```python
from build123d import *

# Parameters (mm, degrees)
EXTRUDE_2_DEPTH     = 70
EXTRUDE_3_DEPTH     = 2
SKETCH_7_W          = 20
SKETCH_7_H          = 18
SKETCH_7_R          = 1.6
EXTRUDE_5_DEPTH     = 4
SKETCH_8_W          = 28
SKETCH_8_H          = 11.5
CUT_EXTRUDE_2_DEPTH = 11.5


with BuildPart() as part:
    # Sketch 1 → Extrude 2 (new body)
    with BuildSketch(Plane.ZY.offset(35)):
        with BuildLine():
            Line((-22.27263006, 25.369984756), (23.72736994, 25.369984756))
            ThreePointArc((23.72736994, 25.369984756), (31.859097923, 22.001712739), (35.22736994, 13.869984756))
            Line((35.22736994, 13.869984756), (35.22736994, 7.291341901))
            ThreePointArc((35.22736994, 7.291341901), (31.859097923, -0.840386083), (23.72736994, -4.208658099))
            Line((23.72736994, -4.208658099), (-22.27263006, -4.208658099))
            ThreePointArc((-22.27263006, -4.208658099), (-30.404358044, -0.840386083), (-33.77263006, 7.291341901))
            Line((-33.77263006, 7.291341901), (-33.77263006, 13.869984756))
            ThreePointArc((-33.77263006, 13.869984756), (-30.404358044, 22.001712739), (-22.27263006, 25.369984756))
        make_face()
        with BuildLine():
            ThreePointArc((-22.27263006, 23.869984756), (-29.343697872, 20.941052568), (-32.27263006, 13.869984756))
            Line((-32.27263006, 13.869984756), (-32.27263006, 7.291341901))
            ThreePointArc((-32.27263006, 7.291341901), (-29.343697872, 0.220274089), (-22.27263006, -2.708658099))
            Line((-22.27263006, -2.708658099), (23.72736994, -2.708658099))
            ThreePointArc((23.72736994, -2.708658099), (30.798437752, 0.220274089), (33.72736994, 7.291341901))
            Line((33.72736994, 7.291341901), (33.72736994, 13.869984756))
            ThreePointArc((33.72736994, 13.869984756), (30.798437752, 20.941052568), (23.72736994, 23.869984756))
            Line((23.72736994, 23.869984756), (-22.27263006, 23.869984756))
        make_face(mode=Mode.SUBTRACT)
    extrude(amount=-EXTRUDE_2_DEPTH)

    # Sketch 1_4 → Extrude 3 (add)
    with BuildSketch(Plane.ZY.offset(35)):
        with BuildLine():
            Line((-22.27263006, 23.869984756), (23.72736994, 23.869984756))
            ThreePointArc((23.72736994, 23.869984756), (30.798437752, 20.941052568), (33.72736994, 13.869984756))
            Line((33.72736994, 13.869984756), (33.72736994, 7.291341901))
            ThreePointArc((33.72736994, 7.291341901), (30.798437752, 0.220274089), (23.72736994, -2.708658099))
            Line((23.72736994, -2.708658099), (-22.27263006, -2.708658099))
            ThreePointArc((-22.27263006, -2.708658099), (-29.343697872, 0.220274089), (-32.27263006, 7.291341901))
            Line((-32.27263006, 7.291341901), (-32.27263006, 13.869984756))
            ThreePointArc((-32.27263006, 13.869984756), (-29.343697872, 20.941052568), (-22.27263006, 23.869984756))
        make_face()
    extrude(amount=-EXTRUDE_3_DEPTH)

    # Sketch 7 → Extrude 5 (add)
    with BuildSketch(Plane(origin=(35, 0, 0), x_dir=(0, 0, -1), z_dir=(1, 0, 0))):
        with Locations((-2.22736994, -11.708658099)):
            Rectangle(SKETCH_7_W, SKETCH_7_H)
        with Locations((4.77263006, -17.708658099)):
            Circle(SKETCH_7_R, mode=Mode.SUBTRACT)
        with Locations((-9.22736994, -17.708658099)):
            Circle(SKETCH_7_R, mode=Mode.SUBTRACT)
    extrude(amount=-EXTRUDE_5_DEPTH)

    # Sketch 8 → Cut-Extrude 2 (cut)
    with BuildSketch(Plane(origin=(0, 0, -33.77263006), x_dir=(-1, 0, 0), z_dir=(0, 0, -1))):
        with Locations((19, 1.541341901)):
            Rectangle(SKETCH_8_W, SKETCH_8_H)
    extrude(amount=-CUT_EXTRUDE_2_DEPTH, mode=Mode.SUBTRACT)


solid = part.part
```
Input: part model. Units: mm. Frame: model coordinates. A direction names the side the tool comes from. Round coordinates to 2 decimals unless told otherwise and drop trailing zeros. Loops run counter-clockwise (first coordinate to the right, second up) from the corner with the lowest first, then second, coordinate; pieces in that order, holes last. Notation, with made-up numbers: (-5, -15) -> (22, -15) arc R20 ccw to (22, 2) -> close; hole circle Ø10 at (-27.75, 8). An arc over 180 degrees is marked (long way). Write each question's results on one line, items separated by ' | '.
1. Section B-B (z = -28.5). Return loops of the section in (x, y).
Geometry results:
outline: (-35, -2.38) -> (-33, -2.38) -> (-33, 21.69) -> (35, 21.69) -> (35, 23.54) -> (-35, 23.54) -> close; (-5, -2.38) -> (35, -2.38) -> (35, -0.53) -> (-5, -0.53) -> close
2. Set-up query: faces 5 (the face through (1, -2.709, 1)), 6 (the face through (33, -13, -7.773)), 7 (the face through (0, 11, -33.773)). Return all of +Z, -Z, +X, -X, +Y, -Y with unobstructed straight access to the full face (end or side cutting, diameter ignored); none if empty.
Geometry results:
face 5: +X | face 6: -Z, +X, -X, -Y | face 7: -Z, +X, -X, +Y, -Y
3. Section A-A (x = 4). Return loops of the section in (y, z), and give its area (3 significant figures).
Geometry results:
outline: (-4.21, -22.27) arc R11.5 ccw to (7.29, -33.77) -> (13.87, -33.77) arc R11.5 ccw to (25.37, -22.27) -> (25.37, 23.73) arc R11.5 ccw to (13.87, 35.23) -> (7.29, 35.23) arc R11.5 ccw to (-4.21, 23.73) -> close; hole (-2.71, -22.27) arc R10 ccw to (7.29, -32.27) -> (13.87, -32.27) arc R10 ccw to (23.87, -22.27) -> (23.87, 23.73) arc R10 ccw to (13.87, 33.73) -> (7.29, 33.73) arc R10 ccw to (-2.71, 23.73) -> close | area: 259 mm2
4. First-contact query: P1, Ø3, axis at x = 2.5, z = 24, coming from the -Y side; P2, Ø1.2, axis at x = 33.5, y = -14.5, coming from the -Z side; P3, Ø14, axis at y = 7, z = 0.5, coming from the +X side. Flat tips, straight axial feed; report the tip coordinate or a pass-through.
Geometry results:
P1: y = -4.21 | P2: z = -7.77 | P3: x = -33
5. Section C-C (y = 2). Return loops of the section in (x, z).
Geometry results:
outline: (-35, -32.48) -> (-33, -32.48) -> (-33, 32.21) -> (35, 32.21) -> (35, 33.94) -> (-35, 33.94) -> close; (-5, -32.48) -> (35, -32.48) -> (35, -30.76) -> (-5, -30.76) -> close
6. Mould query, pull axis Z, two halves, no side actions, for faces 1 (the face through (-33, 10, 0)), 2 (the face through (0.52, 0.14, 30.72)), 3 (the face through (-35, 11, 1)), 4 (the face through (14.72, -0.929, -30.314)). Classes: +Z half, -Z half, draft (parallel to the pull), parting line (faces both ways), or undercut.
Geometry results:
face 1: undercut | face 2: undercut | face 3: draft | face 4: -Z half
7. Section D-D (y = 11). Return loops of the section in (x, z).
Geometry results:
outline: (-35, -33.77) -> (35, -33.77) -> (35, -32.27) -> (-33, -32.27) -> (-33, 33.73) -> (35, 33.73) -> (35, 35.23) -> (-35, 35.23) -> close
8. Ray query, line 1 (Y direction, x = 31.5, z = -5); line 2 (Y direction, x = -19.5, z = -8); line 3 (Z direction, x = 16.5, y = 13). Return the intervals inside material, ascending. Write a range as from..to.
Geometry results:
line 1: -20.71..-19.29, -16.12..-2.71, 23.87..25.37 | line 2: -4.21..-2.71, 23.87..25.37 | line 3: -33.77..-32.27, 33.73..35.23
